Part model, mm, in its own coordinate system. A direction names the side the tool comes from. Give positions to 0.01 mm unless a question says otherwise; leave off trailing zeros. Return JSON: item names as keys, results as strings.
from build123d import *

# Parameters (mm, degrees)
BOSS_EXTRUDE1_DEPTH = 150
WRAP1_START         = 2
WRAP1_DEPTH         = 146
SKETCH5_W           = 52
SKETCH5_H           = 7.004650575
BOSS_EXTRUDE2_DEPTH = 100
SKETCH6_W           = 52
SKETCH6_H           = 6.943317242
CUT_EXTRUDE1_DEPTH  = 48
SKETCH7_R           = 25
CUT_EXTRUDE7_DEPTH  = 2
FILLET1_R           = 10


# Read off the part's stored shape, not the designer's step: Wrap1
with BuildPart() as part:
    # Sketch1 → Boss-Extrude1 (new body)
    with BuildSketch(Plane(origin=(0, 0, 0), x_dir=(1, 0, 0), z_dir=(0, 1, 0))):
        with BuildLine():
            Line((150, 13.582690372), (150, 18.582690372))
            add(Edge.make_bspline(
                [(150, 18.582690372), (0, 28.582690372), (-150, 18.582690372)],
                knots=[0, 0, 0, 1, 1, 1], degree=2))
            Line((-150, 18.582690372), (-150, 13.582690372))
            add(Edge.make_bspline(
                [(150, 13.582690372), (0, 23.582690372), (-150, 13.582690372)],
                knots=[0, 0, 0, 1, 1, 1], degree=2))
        make_face()
    extrude(amount=BOSS_EXTRUDE1_DEPTH)

    # Wrap1 outline → Wrap1 (cut)
    with BuildSketch(Plane(origin=(0, 0, 0), x_dir=(1, 0, 0), z_dir=(0, 1, 0)).offset(WRAP1_START)):
        with BuildLine():
            add(Edge.make_bspline(
                [(-148.024677757, 15.717831092), (-74.012620983, 20.582676475), (1e-09, 22.204328649), (74.012620985, 20.582676475), (148.024677759, 15.717831092)],
                knots=[0.007021667, 0.007021667, 0.007021667, 0.007021667, 0.007021667, 0.992978333, 0.992978333, 0.992978333, 0.992978333, 0.992978333], degree=4))
            Line((-148.024677757, 15.717831092), (-147.89349994, 13.722137634))
            add(Edge.make_bspline(
                [(-147.89349994, 13.722137634), (0, 23.443243111), (147.89349994, 13.722137634)],
                knots=[0.007021667, 0.007021667, 0.007021667, 0.992978333, 0.992978333, 0.992978333], degree=2))
            Line((147.89349994, 13.722137634), (148.024677759, 15.717831092))
        make_face()
    extrude(amount=WRAP1_DEPTH, mode=Mode.SUBTRACT)

    # Sketch5 → Boss-Extrude2 (add)
    with BuildSketch(Plane(origin=(0, 0, 0), x_dir=(1, 0, 0), z_dir=(0, 1, 0))):
        with Locations((0, 26.934793438)):
            Rectangle(SKETCH5_W, SKETCH5_H)
    extrude(amount=BOSS_EXTRUDE2_DEPTH)

    # Sketch6 → Cut-Extrude1 (cut)
    with BuildSketch(Plane.XZ):
        with Locations((0, -26.965460104)):
            Rectangle(SKETCH6_W, SKETCH6_H)
    extrude(amount=-CUT_EXTRUDE1_DEPTH, mode=Mode.SUBTRACT)

    # Sketch7 → Cut-Extrude7 (cut)
    with BuildSketch(Plane(origin=(0, 0, -30.437118725), x_dir=(-1, 0, 0), z_dir=(0, 0, -1))):
        with Locations((0, 74)):
            Circle(SKETCH7_R)
    extrude(amount=-CUT_EXTRUDE7_DEPTH, mode=Mode.SUBTRACT)

    # Fillet1
    fillet1_edges = [part.edges().sort_by_distance(p)[0] for p in [
        (-26, 100, -26.934793437),
        (-26, 48, -26.965460104),
        (26, 48, -26.965460104),
        (26, 100, -26.934793437),
    ]]
    fillet(fillet1_edges, radius=FILLET1_R)


solid = part.part
Q1. 3-axis set-ups, long thin cutter, end or side, ignore diameter. For faces 5 (the flat face through (0, 100, -27)), 6 (the cylindrical face through (-23.15, 96.99, -26.98)), 7 (the cylindrical face through (22.99, 97.15, -26.98)): which of +Z, -Z, +X, -X, +Y, -Y reach the whole face in a straight line?
Established:
{"face 5": "-Z, +X, -X, +Y", "face 6": "-Z, -X, +Y", "face 7": "-Z, +X, +Y"}
Q2. Probe line 1 along Y through (x, z) = (0, -29.15); line 2 along X through (y, z) = (21, -15.25); line 3 along X through (y, z) = (67.5, -25.5). List the from-to ranges inside material, lowest first.
Established:
{"line 1": "y = 48 to 49, 99 to 100", "line 2": "x = -150 to -147.99, 147.99 to 150", "line 3": "x = -26 to 26"}
Q3. Two-plate mould, pull along X, no slides. Class faces 1 (the cylindrical face through (-23.15, 51.01, -26.92)), 2 (the flat face through (0, 48, -27)), 3 (the flat face through (1, 148, -19)), 4 (the flat face through (1, 2, -19)): +X half, -X half, draft (parallel to the pull), parting line (faces both ways), or undercut.
Established:
{"face 1": "-X half", "face 2": "draft", "face 3": "undercut", "face 4": "undercut"}
Q4. Pin check, flat tips, straight feed: pin 1 (15 mm diameter, centred on x = -7, y = 66.5, fed in from -Z); pin 2 (3.5 mm diameter, centred on x = 14.5, z = -15.5, fed in from -Y); pin 3 (2 mm diameter, centred on x = 6, z = -27.5, fed in from -Y); pin 4 (8 mm diameter, centred on y = 81, z = -27.5, fed in from -X). Stop position of each tip, or through.
Established:
{"pin 1": "stops at z = -28.44", "pin 2": "passes through", "pin 3": "stops at y = 48", "pin 4": "stops at x = -26"}
